For this review, use the dimensioned drawing (mm, ordinates from the lowest corner) and the shaded views. Give positions to 0.01 mm unless a question says otherwise; leave off trailing zeros. Order: outer loops, then holes, each group sorted by start corner. A loop starts at its lowest first (then second) coordinate and runs counter-clockwise, first axis right, second up. Notation, with made-up numbers: (70.5, -16) -> (79.5, -16) arc R17 ccw to (79.5, 8) -> close; hole circle Ø11 at (5, 78). An arc over 180 degrees is marked (long way). One line per item, written item: value. Start each with the question number.
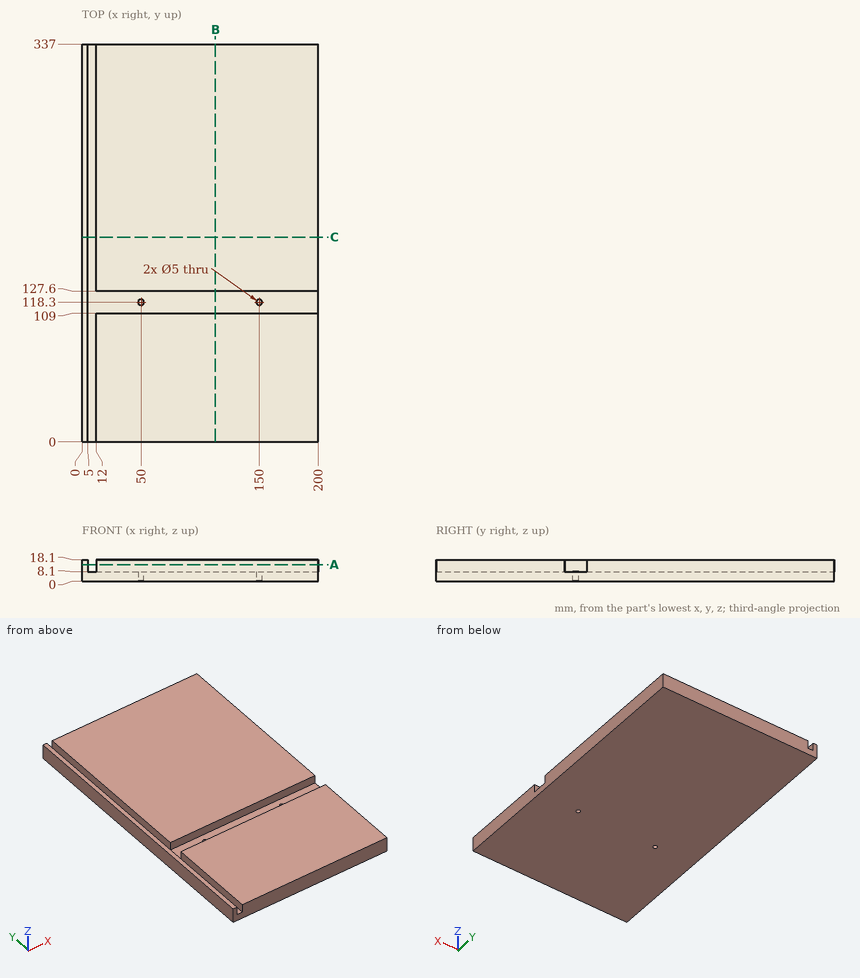
Q1. Take a section at B-B (x = 113). State the section outline as (y, z) points, and give its area (3 significant figures).
Q2. Take a section at C-C (y = 173.5). State the section outline as (x, z) points, and give its area (3 significant figures).
Q3. For pin 1 Ø5 at (x, z) = (89, 13) entering from -Y, flat-tipped, find the tip position at first contact; note if it passes through.
Q4. Take a section at A-A (z = 14). State the section outline as (x, y) points.
Q5. For line 1 along X through (y, z) = (139.5, 16.5); line 2 along X through (y, z) = (118.3, 4.25); line 3 along Y through (x, z) = (50, 5.75), list the stretches that pass through material, from the lowest coordinate up.
Answers below:
1. outline: (0, 0) -> (337, 0) -> (337, 18.1) -> (127.6, 18.1) -> (127.6, 8.1) -> (109, 8.1) -> (109, 18.1) -> (0, 18.1) -> close
1. area: 5,910 mm²
2. outline: (0, 0) -> (200, 0) -> (200, 18.1) -> (12, 18.1) -> (12, 8.1) -> (5, 8.1) -> (5, 18.1) -> (0, 18.1) -> close
2. area: 3,550 mm²
3. pin 1: stops at y = 0
4. outline: (0, 0) -> (5, 0) -> (5, 337) -> (0, 337) -> close; (12, 0) -> (200, 0) -> (200, 109) -> (12, 109) -> close; (12, 127.6) -> (200, 127.6) -> (200, 337) -> (12, 337) -> close
5. line 1: x = 0 to 5, 12 to 200
5. line 2: x = 0 to 47.5, 52.5 to 147.5, 152.5 to 200
5. line 3: y = 0 to 115.8, 120.8 to 337
